from build123d import *

# Parameters (mm, degrees)
SKIZZE1_W                                    = 56
SKIZZE1_H                                    = 86
AUFSATZ_LINEAR_AUSTRAGEN1_DEPTH              = 22
WANDUNG1_T                                   = -2
SKIZZE2_R                                    = 4.5
AUFSATZ_LINEAR_AUSTRAGEN2_DEPTH              = 4
VERRUNDUNG1_R                                = 2
SKIZZE3_W                                    = 22.84
SKIZZE3_H                                    = 14.38
SCHNITT_LINEAR_AUSTRAGEN1_DEPTH              = 2
STIRNSENKUNG_F_R_M3_ZYLINDERSCHRAUBE_2_COUNT = 2
STIRNSENKUNG_F_R_M3_ZYLINDERSCHRAUBE_2_PITCH = 81.987803971
STIRNSENKUNG_F_R_M3_ZYLINDERSCHRAUBE_3_COUNT = 2
STIRNSENKUNG_F_R_M3_ZYLINDERSCHRAUBE_3_PITCH = 71
STIRNSENKUNG_F_R_M3_ZYLINDERSCHRAUBE_4_COUNT = 2
STIRNSENKUNG_F_R_M3_ZYLINDERSCHRAUBE_4_PITCH = 41
SKIZZE7_W                                    = 33.26
SKIZZE7_H                                    = 14.38
SCHNITT_LINEAR_AUSTRAGEN2_DEPTH              = 10
SKIZZE8_W                                    = 39.14
SKIZZE8_H                                    = 9.76
SCHNITT_LINEAR_AUSTRAGEN3_DEPTH              = 10
VERRUNDUNG2_R                                = 3


with BuildPart() as part:
    # Skizze1 → Aufsatz-Linear austragen1 (new body)
    with BuildSketch(Plane(origin=(0, 0, 0), x_dir=(1, 0, 0), z_dir=(0, 1, 0))):
        with Locations((28, 43)):
            Rectangle(SKIZZE1_W, SKIZZE1_H)
    extrude(amount=AUFSATZ_LINEAR_AUSTRAGEN1_DEPTH)

    # Wandung1
    wandung1_openings = [part.faces().sort_by_distance(p)[0] for p in [
        (28, 22, -43),
    ]]
    offset(amount=WANDUNG1_T, openings=wandung1_openings, kind=Kind.INTERSECTION)

    # Skizze2 → Aufsatz-Linear austragen2 (add)
    with BuildSketch(Plane(origin=(0, 2, 0), x_dir=(1, 0, 0), z_dir=(0, 1, 0))):
        with Locations(Location((7.5, 7.5, 0), (0, 0, 90))):
            Circle(SKIZZE2_R)
        with Locations(Location((48.5, 7.5, 0), (0, 0, 90))):
            Circle(SKIZZE2_R)
        with Locations(Location((48.5, 78.5, 0), (0, 0, 90))):
            Circle(SKIZZE2_R)
        with Locations(Location((7.5, 78.5, 0), (0, 0, 90))):
            Circle(SKIZZE2_R)
    extrude(amount=AUFSATZ_LINEAR_AUSTRAGEN2_DEPTH)

    # Verrundung1
    verrundung1_edges = [part.edges().sort_by_distance(p)[0] for p in [
        (0, 11, -86),
        (56, 11, -86),
        (56, 11, 0),
        (0, 11, 0),
    ]]
    fillet(verrundung1_edges, radius=VERRUNDUNG1_R)

    # Skizze3 → Schnitt-Linear austragen1 (cut)
    with BuildSketch(Plane.ZY):
        with Locations((-23, 14.81)):
            Rectangle(SKIZZE3_W, SKIZZE3_H)
    extrude(amount=-SCHNITT_LINEAR_AUSTRAGEN1_DEPTH, mode=Mode.SUBTRACT)

    # Skizze6 → Stirnsenkung für M3 Zylinderschraube mit Innensechskant1 (revolve, cut)
    with BuildSketch(Plane(origin=(48.5, 0, -7.5), x_dir=(0, 0, -1), z_dir=(1, 0, 0))):
        Polygon((0, 0), (0, 15.021463052), (1.7, 14), (1.7, 3.4), (3.25, 3.4), (3.25, 0.025), (3.275, 0), align=None)
    stirnsenkung_f_r_m3_zylinderschraube_mit = revolve(axis=Axis((48.5, -6.35, -7.5), (0, 1, 0)), mode=Mode.SUBTRACT)

    # Stirnsenkung f_r M3 Zylinderschraube 2: Stirnsenkung für M3 Zylinderschraube mit Innensechskant1 ×2
    with Locations(*[Vector(-0.5000743770922673, 0, -0.865982457891487) * (i * STIRNSENKUNG_F_R_M3_ZYLINDERSCHRAUBE_2_PITCH) for i in range(1, STIRNSENKUNG_F_R_M3_ZYLINDERSCHRAUBE_2_COUNT)]):
        add(stirnsenkung_f_r_m3_zylinderschraube_mit, mode=Mode.SUBTRACT)

    # Stirnsenkung f_r M3 Zylinderschraube 3: Stirnsenkung für M3 Zylinderschraube mit Innensechskant1 ×2
    with Locations(*[(0, 0, -i * STIRNSENKUNG_F_R_M3_ZYLINDERSCHRAUBE_3_PITCH) for i in range(1, STIRNSENKUNG_F_R_M3_ZYLINDERSCHRAUBE_3_COUNT)]):
        add(stirnsenkung_f_r_m3_zylinderschraube_mit, mode=Mode.SUBTRACT)

    # Stirnsenkung f_r M3 Zylinderschraube 4: Stirnsenkung für M3 Zylinderschraube mit Innensechskant1 ×2
    with Locations(*[(-i * STIRNSENKUNG_F_R_M3_ZYLINDERSCHRAUBE_4_PITCH, 0, 0) for i in range(1, STIRNSENKUNG_F_R_M3_ZYLINDERSCHRAUBE_4_COUNT)]):
        add(stirnsenkung_f_r_m3_zylinderschraube_mit, mode=Mode.SUBTRACT)

    # Skizze7 → Schnitt-Linear austragen2 (cut)
    with BuildSketch(Plane.ZY):
        with Locations((-55.78, 14.81)):
            Rectangle(SKIZZE7_W, SKIZZE7_H)
    extrude(amount=-SCHNITT_LINEAR_AUSTRAGEN2_DEPTH, mode=Mode.SUBTRACT)

    # Skizze8 → Schnitt-Linear austragen3 (cut)
    with BuildSketch(Plane(origin=(56, 0, 0), x_dir=(0, 0, -1), z_dir=(1, 0, 0))):
        with Locations((43, 14.62)):
            Rectangle(SKIZZE8_W, SKIZZE8_H)
    extrude(amount=-SCHNITT_LINEAR_AUSTRAGEN3_DEPTH, mode=Mode.SUBTRACT)

    # Verrundung2
    verrundung2_edges = [part.edges().sort_by_distance(p)[0] for p in [
        (55, 9.74, -23.43),
        (55, 19.5, -23.43),
        (55, 19.5, -62.57),
        (55, 9.74, -62.57),
    ]]
    fillet(verrundung2_edges, radius=VERRUNDUNG2_R)


solid = part.part
Could you check a few things on this model? Use its own coordinates, in mm. A direction names the side the tool comes from. Round coordinates to 2 decimals unless told otherwise and drop trailing zeros. Loops run counter-clockwise (first coordinate to the right, second up) from the corner with the lowest first, then second, coordinate; pieces in that order, holes last. Notation, with made-up numbers: (-29.5, -24.75) -> (0.5, -24.75) arc R24 ccw to (0.5, -14.75) -> close; hole circle Ø1 at (-19, -0.5). An arc over 180 degrees is marked (long way). Use CSV: the item, a comma, the result in double quotes.
(1) Suppose I cut it at A-A on z = -46. Write out the boundary of the cut face in (x, y).
Return value:
outline,"(0, 0) -> (56, 0) -> (56, 9.74) -> (54, 9.74) -> (54, 2) -> (2, 2) -> (2, 7.62) -> (0, 7.62) -> close; (54, 19.5) -> (56, 19.5) -> (56, 22) -> (54, 22) -> close"
(2) If we mould it in two halves opening along Z, with no side actions, what happens to faces 1 (the flat face through (28, 11, 0)), 2 (the flat face through (56, 8, -42)), 3 (the flat face through (50.4, 6, -78.4)), 4 (the flat face through (1, 15, -11.58))? For each: +Z half, -Z half, draft (parallel to the pull), parting line (faces both ways), or undercut.
Return value:
face 1,"+Z half"
face 2,"draft"
face 3,"undercut"
face 4,"undercut"
(3) For faces 5 (the flat face through (50, 3.4, -77)), 6 (the cylindrical face through (54.99, 10.64, -24.29)), 7 (the flat face through (2, 7, -42)), which set-ups out of +Z, -Z, +X, -X, +Y, -Y let a thin tool reach every point of the face, with its end or its side?
Return value:
face 5,"-Y"
face 6,"+X, -X"
face 7,"+Y"
(4) Suppose I cut it at C-C on x = 48.5. Give the number of separate pieces and of enclosed holes in the cut face, plus the area to 3 significant figures.
Return value:
separate pieces,"3"
enclosed holes,"0"
area,"262 mm²"
(5) Suppose I cut it at B-B on z = -65. Write out the boundary of the cut face in (x, y), plus the area to 3 significant figures.
Return value:
outline,"(0, 0) -> (56, 0) -> (56, 22) -> (54, 22) -> (54, 2) -> (2, 2) -> (2, 7.62) -> (0, 7.62) -> close"
area,"163 mm²"
(6) Suppose I cut it at D-D on y = 11. Write out the boundary of the cut face in (x, z), plus the area to 3 significant figures.
Return value:
outline,"(0, -84) arc R2 ccw to (2, -86) -> (54, -86) arc R2 ccw to (56, -84) -> (56, -62.01) -> (54, -62.01) -> (54, -84) -> (2, -84) -> (2, -72.41) -> (0, -72.41) -> close; (0, -39.15) -> (2, -39.15) -> (2, -34.42) -> (0, -34.42) -> close; (0, -11.58) -> (2, -11.58) -> (2, -2) -> (54, -2) -> (54, -23.99) -> (56, -23.99) -> (56, -2) arc R2 ccw to (54, 0) -> (2, 0) arc R2 ccw to (0, -2) -> close"
area,"360 mm²"
(7) If I drill on probe 1 along X at (y, z) = (4.2, -78.5); probe 2 along X at (y, z) = (1.45, -7.5); probe 3 along Z at (x, y) = (4, 15.5), over which ranges is the centre line in solid material (lowest first)? Write a range as [from, to].
Return value:
probe 1,"x = [0, 2], [3, 5.8], [9.2, 12], [44, 46.8], [50.2, 53], [54, 56]"
probe 2,"x = [0, 4.25], [10.75, 45.25], [51.75, 56]"
probe 3,"z = [-86, -84], [-2, 0]"
(8) Will these pins go through, and if not, where does the flat tip stop? pin 1 Ø1.6 at (x, y) = (0.5, 16) entering from -Z; pin 2 Ø3 at (x, z) = (22, -42.5) entering from +Y; pin 3 Ø2 at (x, z) = (48, -49.5) entering from -Y; pin 4 Ø2 at (x, z) = (8, -8.5) entering from -Y.
Return value:
pin 1,"stops at z = -85.87"
pin 2,"stops at y = 2"
pin 3,"stops at y = 0"
pin 4,"stops at y = 3.4"
